Source: CAD feature listing. Evaluate the final solid. Frame: model axes, mm. A direction names the side the tool comes from. Give positions to 0.01 mm unless a question says otherwise; leave off trailing zeros. Loops run counter-clockwise (first coordinate to the right, second up) from the corner with the lowest first, then second, coordinate; pieces in that order, holes last. Notation, with made-up numbers: (77.25, 74.5) -> (86.25, 74.5) arc R23 cw to (86.25, 90.5) -> close; hole circle Ø9 at (-12, 20.25). An arc over 180 degrees is marked (long way). Put each result on its own line as item: value.
```python
from build123d import *

# Parameters (mm, degrees)
F0_R       = 12.7
F1_DEPTH   = 25.4
F2_W       = 19.4218531251
F2_H       = 8.5854552031
F3_DEPTH   = 63.6221766472
F4_W       = 23.9879162983
F4_H       = 23.1030732393
F1_FACE1_W = 38.1
F1_FACE1_H = 38.1
F5_DEPTH   = 18.6139512807
F6_R       = 2.54
F7_DEPTH   = 25.4
F8_W       = 3.81
F8_H       = 26.416
F9_DEPTH   = 10.4394
F10_W      = 17.78
F10_H      = 25.6636217237
F11_DEPTH  = 20.32
F12_R      = 3.7416241703
F13_DEPTH  = 25.4
F14_W      = 7.112
F14_H      = 51.8768767775
F15_DEPTH  = 10.4394


with BuildPart() as f1:
    # F0 (on Front) → F1 (new body)
    with BuildSketch(Plane.XZ):
        Polygon((42.4058387152, -38.0295165001), (4.3058387152, -38.0295165001), (4.3058387152, -76.1295165001), (42.4058387152, -76.1295165001), (42.4058387152, -57.0795165001), align=None)
        with Locations((29.7058387152, -57.0795165001)):
            Circle(F0_R, mode=Mode.SUBTRACT)
        with Locations((29.7058387152, -57.0795165001)):
            Circle(F0_R)
    extrude(amount=-F1_DEPTH)

    # F2 (on face) → F3 (join)
    with BuildSketch(Plane.XY.offset(-38.0295165001)):
        with Locations((23.6573927104, 21.1072723985)):
            Rectangle(F2_W, F2_H)
    extrude(amount=F3_DEPTH)

    # F4 (on face) + F1_face1 (on face) → F5 (cut)
    with BuildSketch(Plane(origin=(0, 25.4, 0), x_dir=(-1, 0, 0), z_dir=(0, 1, 0))):
        with Locations((-23.0544968509, -56.7404404283)):
            Rectangle(F4_W, F4_H)
    with BuildSketch(Plane(origin=(23.3558387152, 0, -57.0795165001), x_dir=(1, 0, 0), z_dir=(0, -1, 0))):
        Rectangle(F1_FACE1_W, F1_FACE1_H)
    extrude(amount=-F5_DEPTH, dir=(0, 1, 0), mode=Mode.SUBTRACT)

    # F6 (on face) → F7 (cut)
    with BuildSketch(Plane.YZ.offset(33.368319273)):
        with Locations((20.6245447969, 14.7618185729)):
            Circle(F6_R)
    extrude(amount=-F7_DEPTH, mode=Mode.SUBTRACT)

    # F8 (on face) → F9 (join)
    with BuildSketch(Plane(origin=(0, 25.4, 0), x_dir=(-1, 0, 0), z_dir=(0, 1, 0))):
        with Locations((-7.2288869413, -55.5555165001)):
            Rectangle(F8_W, F8_H)
        with Locations((-39.0500968931, -55.5555165001)):
            Rectangle(F8_W, F8_H)
    extrude(amount=F9_DEPTH)

    # F10 (on face) → F11 (join)
    with BuildSketch(Plane.XZ):
        with Locations((23.3558387152, -56.6011555493)):
            Rectangle(F10_W, F10_H)
    extrude(amount=F11_DEPTH)

    # F12 (on face) → F13 (cut)
    with BuildSketch(Plane.YZ.offset(32.2458387152)):
        with Locations((-6.7241610959, -59.7809664111)):
            Circle(F12_R)
    extrude(amount=-F13_DEPTH, mode=Mode.SUBTRACT)

    # F14 (on face) → F15 (join)
    with BuildSketch(Plane(origin=(0, 25.4, 0), x_dir=(-1, 0, 0), z_dir=(0, 1, 0))):
        with Locations((-22.5824661479, -5.3084390238)):
            Rectangle(F14_W, F14_H)
    extrude(amount=F15_DEPTH)


solid = f1.part
```
(1) First-contact query: P1, Ø16.5, axis at y = -8, z = -52.5, coming from the -X side; P2, Ø3, axis at y = 21, z = -12, coming from the -X side; P3, Ø2, axis at x = 24, z = -38.5, coming from the +Y side; P4, Ø1.1, axis at x = 40, y = 31, coming from the -Z side. Flat tips, straight axial feed; report the tip coordinate or a pass-through.
Calculated:
P1: stops at x = 4.31
P2: stops at x = 13.95
P3: stops at y = 25.4
P4: stops at z = -68.76
(2) Draft query along Z for faces 1 (the flat face through (24, 16.815, -7)), 2 (the flat face through (23, 6.786, -57)), 3 (the flat face through (23, 31, 20.63)). Return one class per face: released by +Z, released by -Z, zero draft, split by the parting line, or undercut.
Calculated:
face 1: zero draft
face 2: undercut
face 3: released by +Z
(3) Reachability of faces 4 (the flat face through (37.145, 31, -56)), 5 (the flat face through (39, 31, -68.764)), 6 (the flat face through (7, 31, -42.348)), 7 (the flat face through (40.955, 31, -56)) from +Z, -Z, +X, -X, +Y, -Y: full face, straight path, thin tool, end or side. Return the list, or none.
Calculated:
face 4: +Z, -Z, +Y
face 5: -Z, +X, -X, +Y
face 6: +Z, +X, -X, +Y
face 7: +Z, -Z, +X, +Y
(4) Section A-A on y = 26.5. Return loops of the section in (x, z).
Calculated:
outline: (5.32, -68.76) -> (9.13, -68.76) -> (9.13, -42.35) -> (5.32, -42.35) -> close; (19.03, -31.25) -> (26.14, -31.25) -> (26.14, 20.63) -> (19.03, 20.63) -> close; (37.15, -68.76) -> (40.96, -68.76) -> (40.96, -42.35) -> (37.15, -42.35) -> close
(5) Line query: probe 1 along Y at (x, z) = (24, 15); probe 2 along X at (y, z) = (11, -60); probe 3 along Z at (x, y) = (36, 23.5). Output: solid intervals per line, ascending. Write a range as from..to.
Calculated:
probe 1: y = 16.81..18.1, 23.15..35.84
probe 2: x = 4.31..11.06, 35.05..42.41
probe 3: z = -76.13..-38.03
(6) Section D-D on z = -12. Return loops of the section in (x, y).
Calculated:
outline: (13.95, 16.81) -> (33.37, 16.81) -> (33.37, 25.4) -> (26.14, 25.4) -> (26.14, 35.84) -> (19.03, 35.84) -> (19.03, 25.4) -> (13.95, 25.4) -> close
(7) Section C-C on x = 22.5. Return loops of the section in (y, z), then the cut area to 3 significant figures.
Calculated:
outline: (-20.32, -69.43) -> (0, -69.43) -> (0, -76.13) -> (25.4, -76.13) -> (25.4, -68.29) -> (6.79, -68.29) -> (6.79, -45.19) -> (25.4, -45.19) -> (25.4, -31.25) -> (35.84, -31.25) -> (35.84, 20.63) -> (25.4, 20.63) -> (25.4, 25.59) -> (16.81, 25.59) -> (16.81, -38.03) -> (0, -38.03) -> (0, -43.77) -> (-20.32, -43.77) -> close; hole circle Ø7.48 at (-6.72, -59.78); hole circle Ø5.08 at (20.62, 14.76)
area: 2,080 mm²
(8) Section B-B on y = 12. Return loops of the section in (x, z).
Calculated:
outline: (4.31, -76.13) -> (42.41, -76.13) -> (42.41, -38.03) -> (4.31, -38.03) -> close; hole (11.06, -68.29) -> (35.05, -68.29) -> (35.05, -45.19) -> (11.06, -45.19) -> close
